Could you check a few things on this model? Use its own coordinates, in mm. Coordinates: 2 decimals unless noted, no trailing zeros. Loops run counter-clockwise (first coordinate to the right, second up) from the corner with the lowest first, then second, coordinate; pieces in that order, holes last. Notation, with made-up numbers: (30, 87) - (69, 87) arc R27 ccw to (69, 114) - close; hole circle Ø4 at (61.5, 25). An arc over 180 degrees is marked (long way). Use CSV: the item, a comma, the result in double quotes.
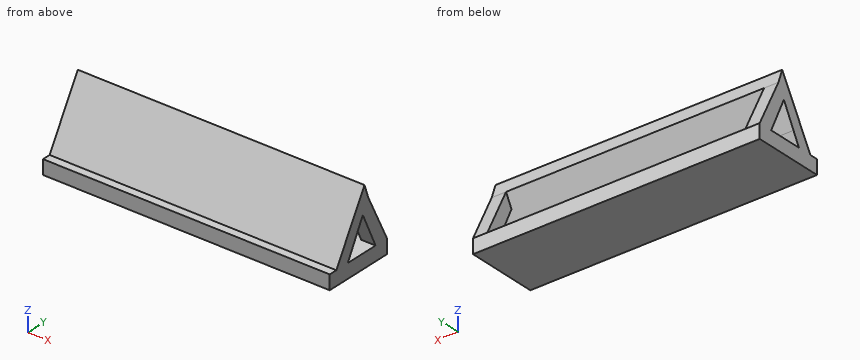
from build123d import *

# Parameters (mm, degrees)
F0_W      = 50.8
F0_H      = 12.7
F1_DEPTH  = 2.54
F3_DEPTH  = 50.8
F5_DEPTH  = 50.8
F7_DEPTH  = 50.8
F8_R      = 0.7792520308
F9_DEPTH  = 25.4
F11_DEPTH = 50.8
F13_W     = 2.54
F13_H     = 2.54
F12_W     = 2.54
F12_H     = 2.54
F16_W     = 2.54
F16_H     = 2.54
F15_W     = 2.54
F15_H     = 2.54


with BuildPart() as f1:
    # F0 (on Top) → F1 (new body)
    with BuildSketch(Plane.XY):
        with Locations((25.4, 6.35)):
            Rectangle(F0_W, F0_H)
    extrude(amount=F1_DEPTH)

    # F2 (on Right) → F3 (join)
    with BuildSketch(Plane.YZ):
        Polygon((7.7083574152, 13.351266686), (0, 0), (12.3911025003, 0), align=None)
    extrude(amount=F3_DEPTH)

    # F4 (on face) → F5 (cut)
    with BuildSketch(Plane.YZ.offset(50.8)):
        Polygon((8.549014916, 10.9544156338), (4.0064696837, 2.54), (11.5002377759, 2.54), align=None)
    extrude(amount=-F5_DEPTH, mode=Mode.SUBTRACT)



with BuildPart() as f7:
    # F6 (on face) → F7 (new body)
    with BuildSketch(Plane.YZ.offset(50.8)):
        Polygon((5.2130930665, 4.775097316), (4.0064696837, 2.54), (6.5464696837, 2.54), align=None)
    extrude(amount=-F7_DEPTH)


with BuildPart() as f1_1:
    add(f1.part)

    add(f7.part)  # F9 merges F7
    # F8 (on face) → F9 (join)
    with BuildSketch(Plane.YZ.offset(50.8)):
        with Locations((4.0064696837, 2.54)):
            Circle(F8_R)
    extrude(amount=-F9_DEPTH)

    # F10 (on face) → F11 (cut)
    with BuildSketch(Plane.YZ.offset(50.8)):
        Polygon((4.0064696837, 2.54), (6.5464696837, 2.54), (5.2130930665, 4.775097316), align=None)
    extrude(amount=-F11_DEPTH, mode=Mode.SUBTRACT)

    # F13 (on face) → F14 section 0
    with BuildSketch(Plane(origin=(0, 2.0405452679, -1.1015939289), x_dir=(-1, 0, 0), z_dir=(0, 0.8799595732, -0.4750485759))):
        with Locations((-49.53, 12.4306402674)):
            Rectangle(F13_W, F13_H)
    # F12 (on face) → F14 section 1
    with BuildSketch(Plane.XY.offset(2.54)):
        with Locations((49.53, 11.43)):
            Rectangle(F12_W, F12_H)
    loft()

    # F16 (on face) → F17 section 0
    with BuildSketch(Plane(origin=(0, 2.0405452679, -1.1015939289), x_dir=(-1, 0, 0), z_dir=(0, 0.8799595732, -0.4750485759))):
        with Locations((-1.27, 12.4306402674)):
            Rectangle(F16_W, F16_H)
    # F15 (on face) → F17 section 1
    with BuildSketch(Plane.XY.offset(2.54)):
        with Locations((1.27, 11.43)):
            Rectangle(F15_W, F15_H)
    loft()


solid = f1_1.part
(1) Suppose I cut it at B-B (x = 38.5). Write out the boundary of the cut face in (y, z), plus the area to 3 significant figures.
Computed:
outline,"(0, 0) - (12.7, 0) - (12.7, 2.54) - (4.01, 2.54) - (8.55, 10.95) - (7.71, 13.35) - (1.47, 2.54) - (0, 2.54) - close"
area,"55.0 mm²"
(2) Suppose I cut it at A-A (y = 4.5). Write out the boundary of the cut face in (x, z), plus the area to 3 significant figures.
Computed:
outline,"(0, 0) - (50.8, 0) - (50.8, 2.54) - (0, 2.54) - close; (0, 3.45) - (50.8, 3.45) - (50.8, 7.79) - (0, 7.79) - close"
area,"350 mm²"
(3) Suppose I cut it at C-C (z = 7.5). State how many separate pieces and enclosed holes the cut face has, plus the area to 3 significant figures.
Computed:
separate pieces,"3"
enclosed holes,"0"
area,"132 mm²"
(4) Will these pins go through, and if not, where does the flat tip stop? pin 1 (2 mm diameter, centred on x = 26.5, z = 8, fed in from +Y); pin 2 (5 mm diameter, centred on x = 17, z = 8.5, fed in from -Y); pin 3 (3 mm diameter, centred on x = 6.5, y = 7.5, fed in from +Z).
Computed:
pin 1,"stops at y = 7.49"
pin 2,"stops at y = 3.46"
pin 3,"stops at z = 13.35"
(5) Please list where these lines run through material, in increasing order: line 1 (X direction, y = 10.25, z = 4); line 2 (Z direction, x = 28.5, y = 1.25); line 3 (Z direction, x = 7.5, y = 5.25).
Computed:
line 1,"x = 0 to 2.54, 48.26 to 50.8"
line 2,"z = 0 to 2.54"
line 3,"z = 0 to 2.54, 4.84 to 9.09"
